Can you work these out from the model? Positions are in its coordinate system, mm. A direction names the side the tool comes from. Give positions to 0.01 mm unless a question says otherwise; leave off trailing zeros. Loops run counter-clockwise (first coordinate to the right, second up) from the corner with the lowest first, then second, coordinate; pieces in that order, holes last. Notation, with made-up numbers: M 52.25,-35.5 L 111.25,-35.5 A23 cw 111.25,-9.5 Z; hole C 89.5,-12.75 d3. An arc over 180 degrees is marked long. Put each result on its own line as item: value. Start each with the question number.
1) Please list where these lines run through material, in increasing order: line 1 along Y through (x, z) = (2, -6.5); line 2 along Z through (x, y) = (-14, 3.25); line 3 along Z through (x, y) = (12, 9.25). Write a range as from..to.
2) Imagine slicing it at B-B (y = 4.5). Write out the boundary of the cut face in (x, z) (3 decimals), then the cut area to 3 significant figures.
3) For faces 1 (the flat face through (0, 0, 5)), 2 (the flat face through (0, 2.54, -2)), which set-ups out of +Z, -Z, +X, -X, +Y, -Y let a thin tool reach every point of the face, with its end or its side?
4) If we mould it in two halves opening along Z, with no side actions, what happens to faces 3 (the conical face through (-16.775, 8.255, 12.862)), 4 (the flat face through (0, 12.7, 0)), 5 (the flat face through (0, 11.112, -10)), 6 (the flat face through (0, 6, -1.397))? For each: +Z half, -Z half, draft (parallel to the pull), parting line (faces both ways), or undercut.
5) For P1, Ø1.7, axis at x = -0.5, y = 5.5, coming from the +Z side; P2, Ø3.5, axis at x = -2, z = -12, coming from the +Y side; P3, Ø6, axis at x = 4.5, z = -12.5, coming from the +Y side; P4, Ø5, axis at x = 0, z = 0, coming from the -Y side, each with a flat end and sliding along its axis, tell me the tip position at first contact or that it passes through.
6) Imagine slicing it at A-A (y = 8.5). Write out the boundary of the cut face in (x, z) (3 decimals).
from build123d import *

# Parameters (mm, degrees)
SKETCH1_R           = 22.225
BOSS_EXTRUDE1_DEPTH = 12.7
BOSS_EXTRUDE1_TAPER = 7.5
FILLET1_R           = 1.5875
SKETCH2_R           = 6.35
CUT_EXTRUDE1_DEPTH  = 1.5875
FILLET2_R           = 0.79375
CUT_EXTRUDE2_DEPTH  = 9.525
SKETCH4_R           = 3.175
CUT_EXTRUDE3_DEPTH  = 2.54


with BuildPart() as part:
    # Sketch1 → Boss-Extrude1 (new body)
    with BuildSketch(Plane(origin=(0, 0, 0), x_dir=(1, 0, 0), z_dir=(0, 1, 0))):
        Circle(SKETCH1_R)
    extrude(amount=BOSS_EXTRUDE1_DEPTH, taper=BOSS_EXTRUDE1_TAPER)

    # Fillet1
    fillet1_edges = [part.edges().sort_by_distance(p)[0] for p in [
        (-20.553013281, 12.7, 0),
    ]]
    fillet(fillet1_edges, radius=FILLET1_R)

    # Sketch2 → Cut-Extrude1 (cut)
    with BuildSketch(Plane(origin=(0, 12.7, 0), x_dir=(1, 0, 0), z_dir=(0, 1, 0))):
        with Locations(Location((0, 9.580406573, 0), (0, 0, 270))):
            Circle(SKETCH2_R)
    extrude(amount=-CUT_EXTRUDE1_DEPTH, mode=Mode.SUBTRACT)

    # Fillet2
    fillet2_edges = [part.edges().sort_by_distance(p)[0] for p in [
        (0, 11.1125, -15.930406573),
        (0, 12.7, -15.930406573),
    ]]
    fillet(fillet2_edges, radius=FILLET2_R - 0.0001)  # a hair under: the kernel refuses the full size

    # Sketch3 → Cut-Extrude2 (cut)
    with BuildSketch(Plane.XZ):
        with BuildLine():
            Line((-2.851142929, -1.397), (2.851142929, -1.397))
            ThreePointArc((2.851142929, -1.397), (0, 3.175), (-2.851142929, -1.397))
        make_face()
    extrude(amount=-CUT_EXTRUDE2_DEPTH, mode=Mode.SUBTRACT)

    # Sketch4 → Cut-Extrude3 (cut)
    with BuildSketch(Plane.XZ):
        with Locations(Location((0, 0, 0), (0, 0, 270))):
            Circle(SKETCH4_R)
    extrude(amount=-CUT_EXTRUDE3_DEPTH, mode=Mode.SUBTRACT)


solid = part.part
Recorded:
1. line 1: 0..11.11
1. line 2: -16.71..16.71
1. line 3: -17.24..17.24
2. outline: C 0,0 d43.265; hole M -2.851,-1.397 L 2.851,-1.397 A3.175 ccw long Z
2. area: 1,450 mm²
3. face 1: +Z, -Z, +X, -X, -Y
3. face 2: -Y
4. face 3: parting line
4. face 4: draft
4. face 5: undercut
4. face 6: undercut
5. P1: z = 21.61
5. P2: y = 11.11
5. P3: y = 12.7
5. P4: y = 2.54
6. outline: C 0,0 d42.212; hole M -2.851,-1.397 L 2.851,-1.397 A3.175 ccw long Z
